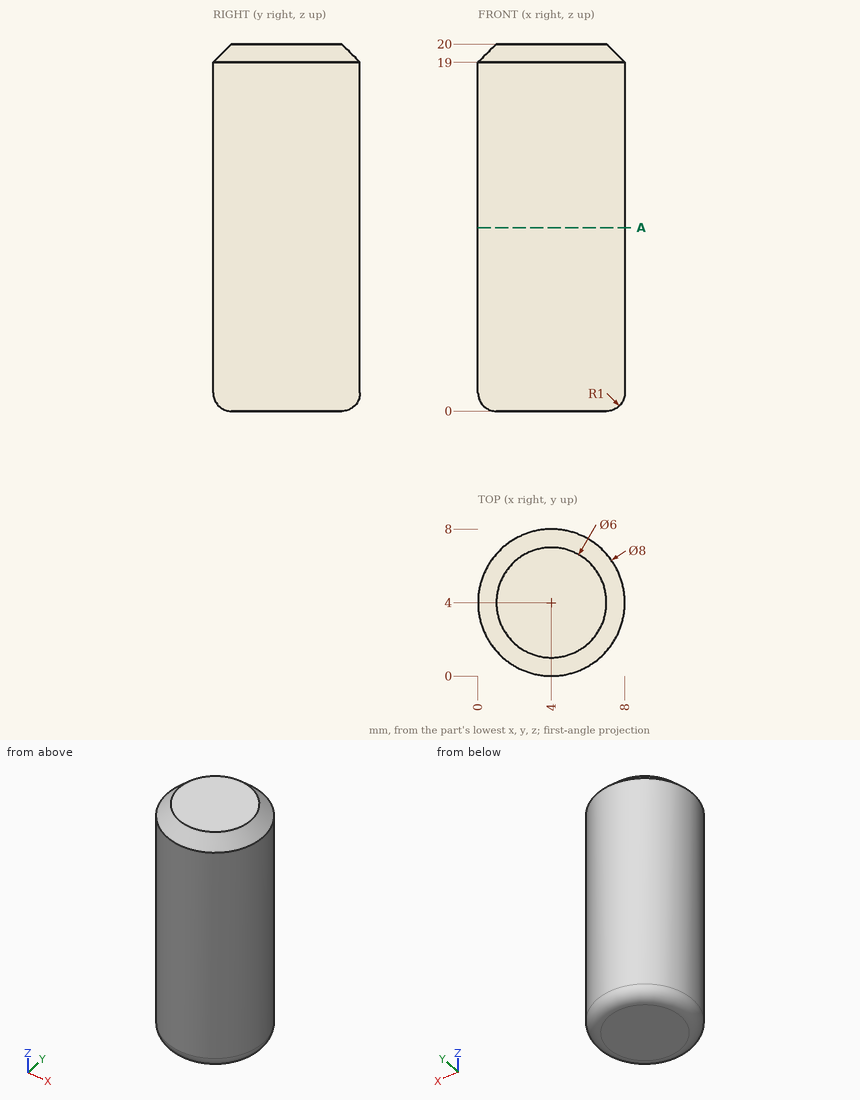
Check sheet for the drawn part. Datum: minimum x, y, z corner. Units: mm. Coordinates: 2 decimals unless noted, no trailing zeros. Write each loop counter-clockwise with the first axis right and the second up, starting at its lowest first coordinate (ties: lowest second). Pieces come first, ordered by that corner, then holes. Notation, with made-up numbers: (29, 24.25) - (38, 24.25) arc R29 cw to (38, 50.25) - close; hole circle Ø4 at (-29, -0.75). An arc over 180 degrees is marked (long way). Answer as a JSON object with one key per item and string values.
(1) Gauge pin test, flat ends, axial feed: pin 1 Ø1.5 at (x, z) = (2.5, 14) entering from +Y; pin 2 Ø1 at (x, z) = (5.5, 3.5) entering from -Y. Record the tip position at first contact, or that the pin passes through.
Report:
{"pin 1": "y = 7.93", "pin 2": "y = 0.13"}
(2) Thickness scan on line 1 along Z through (x, y) = (7.75, 4.5); line 2 along Z through (x, y) = (7, 4.5); line 3 along Y through (x, z) = (6.75, 12.75). Record the ranges inside material, lowest first.
Report:
{"line 1": "0.38 to 19.22", "line 2": "0 to 19.96", "line 3": "1.1 to 6.9"}
(3) Cross-section at A-A on z = 10. Record the cut outline in (x, y).
Report:
{"outline": "circle Ø8 at (4, 4)"}
